Can you work these out from the model? Positions are in its coordinate system, mm. Face numbers are marked on the shaded views. A direction names the side the tool comes from. Round coordinates to 2 decimals unless told otherwise and drop trailing zeros. Write each loop counter-clockwise with the first axis right and the second up, starting at its lowest first coordinate (ties: lowest second). Pieces come first, ordered by that corner, then holes. Notation, with made-up numbers: M 53,-9.75 L 63,-9.75 A26 cw 63,29.25 Z; hole C 21,76.25 d2. An arc over 180 degrees is marked long. Answer as a JSON object with one key per item and string values. Group by question number.
1) On a 3-axis mill with a long thin cutter (end or side, diameter ignored), from which of +Z, -Z, +X, -X, +Y, -Y can I reach the whole of each face in a straight line? I mean the marked faces 1 and 2. Say none if no direction works.
2) Suppose I cut it at D-D, the plane z = 40. Write out the boundary of the cut face in (x, y), and give its area (3 significant figures).
3) Please list where these lines run through material, in increasing order: L1, parallel to Y at x = 0, z = 2.6; L2, parallel to Y at x = 0, z = 1; L3, parallel to Y at x = 10.5, z = 6. Write a range as [from, to].
4) If we mould it in two halves opening along X, with no side actions, what happens to the marked faces 3, 4 and 5? For each: +X half, -X half, draft (parallel to the pull), parting line (faces both ways), or undercut.
5) I'm going to push flat-ended pins straight in: pin 1 Ø0.8 at (y, z) = (6, 18.5) entering from +X; pin 2 Ø3 at (x, y) = (-13.5, 0) entering from -Z; pin 3 Ø5 at (y, z) = (-7.5, 22) entering from +X (3 decimals); pin 4 Ø8 at (y, z) = (4.5, 26) entering from -X. Where does each tip first touch, or does it pass through?
6) Suppose I cut it at B-B, the plane z = 14.5. Write out the boundary of the cut face in (x, y), and give its area (3 significant figures).
7) Suppose I cut it at A-A, the plane y = 0. State how many separate pieces and enclosed holes the cut face has, and give its area (3 significant figures).
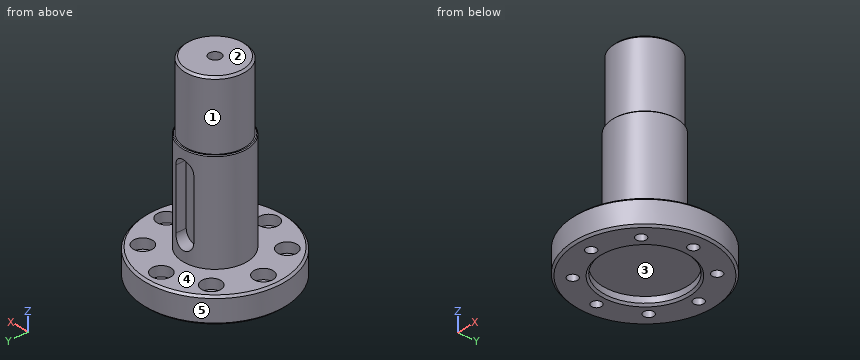
from build123d import *

# Parameters (mm, degrees)
SKETCH_1_R          = 17.5
SKETCH_1_R_2        = 1.25
EXTRUDE_1_DEPTH     = 6.4
SKETCH_2_R          = 8
EXTRUDE_2_DEPTH     = 42
CUT_EXTRUDE_1_DEPTH = 3
SKETCH_11_R         = 1.5
CUT_EXTRUDE_4_DEPTH = 5
SKETCH_12_OUTSIDE_W = 50.846
SKETCH_12_OUTSIDE_H = 50.846
SKETCH_12_OUTSIDE_R = 7.5
CUT_EXTRUDE_5_DEPTH = 17
CHAMFER_1_SIZE      = 0.5
CHAMFER_2_SIZE      = 0.2
SKETCH_39_R         = 2.4
CUT_EXTRUDE_8_DEPTH = 2.5
CHAMFER_3_SIZE      = 0.5
SKETCH_40_R         = 10.5
CUT_EXTRUDE_9_DEPTH = 2
CHAMFER_4_SIZE      = 0.5


with BuildPart() as part:
    # 草图1 → 凸台-拉伸1 (new body)
    with BuildSketch(Plane.XY):
        Circle(SKETCH_1_R)
        with Locations((0, 13.5)):
            Circle(SKETCH_1_R_2, mode=Mode.SUBTRACT)
        with Locations((9.545941546, 9.545941546)):
            Circle(SKETCH_1_R_2, mode=Mode.SUBTRACT)
        with Locations((13.5, 0)):
            Circle(SKETCH_1_R_2, mode=Mode.SUBTRACT)
        with Locations((9.545941546, -9.545941546)):
            Circle(SKETCH_1_R_2, mode=Mode.SUBTRACT)
        with Locations((0, -13.5)):
            Circle(SKETCH_1_R_2, mode=Mode.SUBTRACT)
        with Locations((-9.545941546, -9.545941546)):
            Circle(SKETCH_1_R_2, mode=Mode.SUBTRACT)
        with Locations((-13.5, 0)):
            Circle(SKETCH_1_R_2, mode=Mode.SUBTRACT)
        with Locations((-9.545941546, 9.545941546)):
            Circle(SKETCH_1_R_2, mode=Mode.SUBTRACT)
    extrude(amount=EXTRUDE_1_DEPTH)

    # 草图2 → 凸台-拉伸2 (add)
    with BuildSketch(Plane.XY.offset(6.4)):
        with Locations(Location((0, 0, 0), (0, 0, 180))):
            Circle(SKETCH_2_R)
    extrude(amount=EXTRUDE_2_DEPTH)

    # 草图6 → 切除-拉伸1 (cut)
    with BuildSketch(Plane(origin=(0, 8, 0), x_dir=(1, 0, 0), z_dir=(0, 1, 0))):
        with BuildLine():
            Line((-2.5, -11.4), (-2.5, -26.4))
            ThreePointArc((-2.5, -26.4), (0, -28.9), (2.5, -26.4))
            Line((2.5, -26.4), (2.5, -11.4))
            ThreePointArc((2.5, -11.4), (0, -8.9), (-2.5, -11.4))
        make_face()
    extrude(amount=-CUT_EXTRUDE_1_DEPTH, mode=Mode.SUBTRACT)

    # 草图11 → 切除-拉伸4 (cut)
    with BuildSketch(Plane.XY.offset(48.4)):
        Circle(SKETCH_11_R)
    extrude(amount=-CUT_EXTRUDE_4_DEPTH, mode=Mode.SUBTRACT)

    # 草图12 outside → 切除-拉伸5 (cut)
    with BuildSketch(Plane.XY.offset(48.4)):
        Rectangle(SKETCH_12_OUTSIDE_W, SKETCH_12_OUTSIDE_H)
        Circle(SKETCH_12_OUTSIDE_R, mode=Mode.SUBTRACT)
    extrude(amount=-CUT_EXTRUDE_5_DEPTH, mode=Mode.SUBTRACT)

    # 倒角1
    chamfer_1_edges = [part.edges().sort_by_distance(p)[0] for p in [
        (-7.5, 0, 48.4),
    ]]
    chamfer(chamfer_1_edges, length=CHAMFER_1_SIZE)

    # 倒角2
    chamfer_2_edges = [part.edges().sort_by_distance(p)[0] for p in [
        (8, 0, 31.4),
    ]]
    chamfer(chamfer_2_edges, length=CHAMFER_2_SIZE)

    # 草图39 → 切除-拉伸8 (cut)
    with BuildSketch(Plane.XY.offset(6.4)):
        with Locations((-9.545941546, 9.545941546)):
            Circle(SKETCH_39_R)
        with Locations((0, 13.5)):
            Circle(SKETCH_39_R)
        with Locations((9.545941546, 9.545941546)):
            Circle(SKETCH_39_R)
        with Locations((13.5, 0)):
            Circle(SKETCH_39_R)
        with Locations((9.545941546, -9.545941546)):
            Circle(SKETCH_39_R)
        with Locations((0, -13.5)):
            Circle(SKETCH_39_R)
        with Locations((-9.545941546, -9.545941546)):
            Circle(SKETCH_39_R)
        with Locations((-13.5, 0)):
            Circle(SKETCH_39_R)
    extrude(amount=-CUT_EXTRUDE_8_DEPTH, mode=Mode.SUBTRACT)

    # 倒角3
    chamfer_3_edges = [part.edges().sort_by_distance(p)[0] for p in [
        (-17.5, 0, 0),
        (-17.5, 0, 6.4),
    ]]
    chamfer(chamfer_3_edges, length=CHAMFER_3_SIZE)

    # 草图40 → 切除-拉伸9 (cut)
    with BuildSketch(Plane(origin=(0, 0, 0), x_dir=(-1, 0, 0), z_dir=(0, 0, -1))):
        Circle(SKETCH_40_R)
    extrude(amount=-CUT_EXTRUDE_9_DEPTH, mode=Mode.SUBTRACT)

    # 倒角4
    chamfer_4_edges = [part.edges().sort_by_distance(p)[0] for p in [
        (10.5, 0, 0),
    ]]
    chamfer(chamfer_4_edges, length=CHAMFER_4_SIZE)


solid = part.part
Results:
{
 "1": {"face 1": "+Z", "face 2": "+Z, +X, -X, +Y, -Y"},
 "2": {"outline": "C 0,0 d15", "area": "177 mm^2"},
 "3": {"L1": "[-17.5, -14.75], [-12.25, 12.25], [14.75, 17.5]", "L2": "[-17.5, -14.75], [-12.25, -10.5], [10.5, 12.25], [14.75, 17.5]", "L3": "[-13.87, -11.75], [-7.34, 7.34], [11.75, 13.87]"},
 "4": {"face 3": "undercut", "face 4": "draft", "face 5": "parting line"},
 "5": {"pin 1": "x = 5.71", "pin 2": "z = 0", "pin 3": "x = 6.245", "pin 4": "x = -7.98"},
 "6": {"outline": "M -2.5,5 L -2.5,7.6 A8 ccw long 2.5,7.6 L 2.5,5 Z", "area": "187 mm^2"},
 "7": {"separate pieces": "3", "enclosed holes": "0", "area": "777 mm^2"}
}
